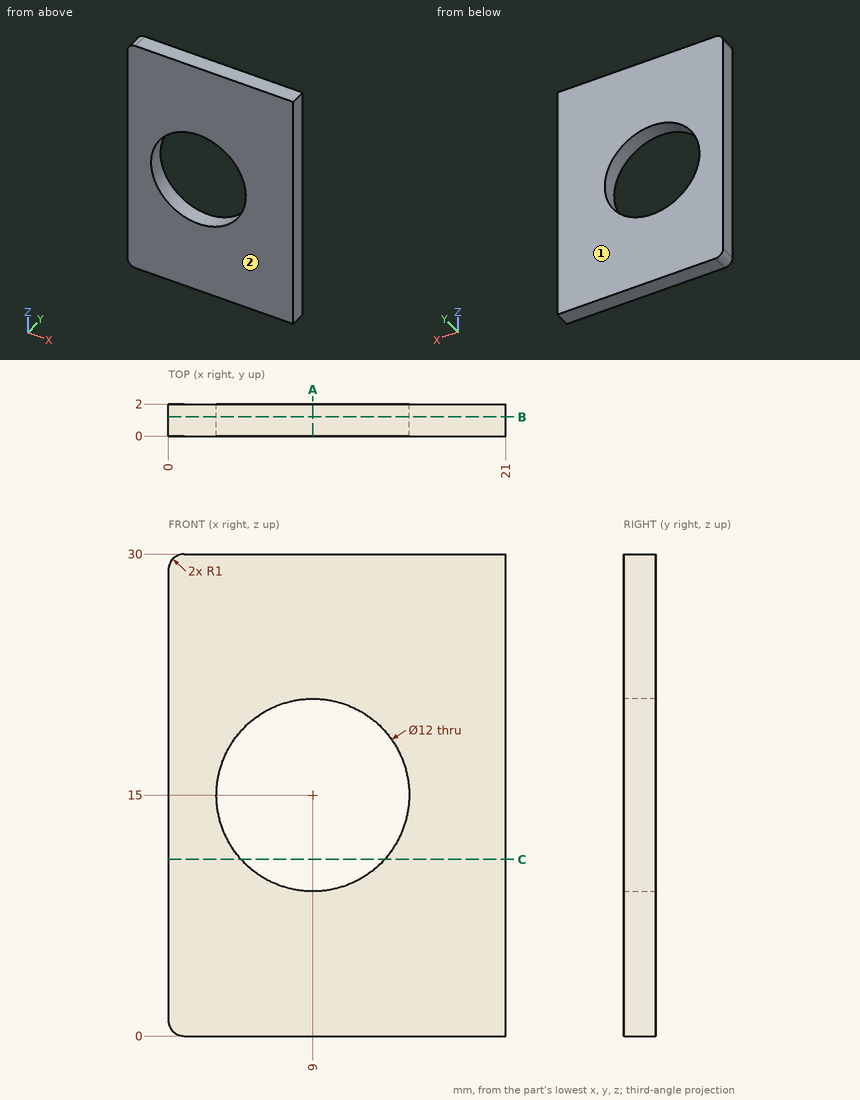
Geometry check sheet. Reference: drawing and pictorial views, mm from the part's lowest x, y, z. Coordinates: 2 decimals unless noted, no trailing zeros. Loops run counter-clockwise (first coordinate to the right, second up) from the corner with the lowest first, then second, coordinate; pieces in that order, holes last.
1) Release check for a two-part mould opening along Y. For the marked faces 1 and 2 record: released by +Y, released by -Y, zero draft, split by the parting line, or undercut.
2) Sectioned sample at A-A (x = 9). Record the boundary of the cut face in (y, z).
3) Sectioned sample at C-C (z = 11). Record the boundary of the cut face in (x, y), and give its area (3 significant figures).
4) Sectioned sample at B-B (y = 1.2). Record the boundary of the cut face in (x, z), and give its area (3 significant figures).
5) Material ranges on probe 1 along X at (y, z) = (0.9, 15); probe 2 along Z at (x, y) = (3.5, 1.55); probe 3 along X at (y, z) = (0.8, 12.75), recorded low to high.
Check sheet entries:
1. face 1: released by +Y
1. face 2: released by -Y
2. outline: (0, 0) - (2, 0) - (2, 9) - (0, 9) - close; (0, 21) - (2, 21) - (2, 30) - (0, 30) - close
3. outline: (0, 0) - (4.53, 0) - (4.53, 2) - (0, 2) - close; (13.47, 0) - (21, 0) - (21, 2) - (13.47, 2) - close
3. area: 24.1 mm2
4. outline: (0, 1) arc R1 ccw to (1, 0) - (21, 0) - (21, 30) - (1, 30) arc R1 ccw to (0, 29) - close; hole circle Ø12 at (9, 15)
4. area: 516 mm2
5. probe 1: x = 0 to 3, 15 to 21
5. probe 2: z = 0 to 12.6, 17.4 to 30
5. probe 3: x = 0 to 3.44, 14.56 to 21
